from build123d import *

# Parameters (mm, degrees)
F1_DEPTH = 50
F3_DEPTH = 25
F4_R     = 4.5
F5_DEPTH = 25


with BuildPart() as f1:
    # F0 (on Top) → F1 (new body)
    with BuildSketch(Plane.XY):
        Polygon((1.597207, 5.6), (-2.124833, 5.6), (-4.124833, 5.6), (-4.124833, -6.4), (-2.124833, -6.4), (1.597207, -6.4), (3.597207, -6.4), (3.597207, 5.6), align=None)
        Polygon((-0.528539, 3), (-0.528539, 4), (0.471461, 4), (0.471461, 3), (1.597207, 3), (1.597207, -3.9), (0.471461, -3.9), (0.471461, -4.4), (-0.528539, -4.4), (-0.528539, -3.9), (-2.124833, -3.9), (-2.124833, 3), align=None, mode=Mode.SUBTRACT)
    extrude(amount=F1_DEPTH)

    # F2 (on face) → F3 (cut)
    with BuildSketch(Plane.YZ.offset(3.597207)):
        with BuildLine():
            Line((-3.9, 29.523588), (-3.9, 20.935996))
            ThreePointArc((-3.9, 20.935996), (-0.366142, 17.178962), (3.6, 20.476412))
            Line((3.6, 20.476412), (3.6, 29.064004))
            ThreePointArc((3.6, 29.064004), (0.066142, 32.821038), (-3.9, 29.523588))
        make_face()
    extrude(amount=-F3_DEPTH, mode=Mode.SUBTRACT)

    # F4 (on face) → F5 (cut)
    with BuildSketch(Plane(origin=(-4.124833, 0, 0), x_dir=(0, -1, 0), z_dir=(-1, 0, 0))):
        with Locations((0, 50)):
            Circle(F4_R)
    extrude(amount=-F5_DEPTH, mode=Mode.SUBTRACT)


solid = f1.part
Could you check a few things on this model? Use its own coordinates, in mm. A direction names the side the tool comes from. Give positions to 0.01 mm unless a question says otherwise; leave off trailing zeros. Loops run counter-clockwise (first coordinate to the right, second up) from the corner with the lowest first, then second, coordinate; pieces in that order, holes last. Notation, with made-up numbers: (-21.5, 22) -> (32.5, 22) arc R13 ccw to (32.5, 47) -> close; hole circle Ø10 at (-12, -28). An arc over 180 degrees is marked (long way). Answer as CSV lines item,"result". Start each with the question number.
(1) We'd pull the mould along Y, two halves only. Please class faces 6 (the flat face through (3.597, -4.5, 24.6)), 7 (the flat face through (0, -6.4, 25)), 8 (the flat face through (0, -4.4, 24)): released by +Y, released by -Y, zero draft, split by the parting line, or undercut.
(2) Which directions (+Z, -Z, +X, -X, +Y, -Y) give clear straight access to the entire face, cutting with the end or side of a thin tool? Please do faces 1 (the flat face through (0, 5, 50)), 2 (the flat face through (-4.125, 4, 25)), 3 (the cylindrical face through (2.404, 0.145, 32.815)), 4 (the flat face through (1, -3.9, 24)), 5 (the flat face through (1, 3, 9)).
(3) If we section it at C-C on z = 33.5: Write out the boundary of the cut face in (x, y).
(4) I need wall thicknesses on probe 1 along Y at (x, z) = (-1.75, 40); probe 2 along X at (y, z) = (-1, 11); probe 3 along Y at (x, z) = (-1.25, 29). Which ranges of each line are inside material? Lowest first, please.
(5) If we section it at B-B on x = -1: Write out the boundary of the cut face in (y, z) (3 decimals).
(6) If we section it at A-A on z = 25.5: Write out the boundary of the cut face in (x, y), then the cut area to 3 significant figures.
(7) If we section it at D-D on x = -3: Write out the boundary of the cut face in (y, z), then the cut area to 3 significant figures.
Computed:
1,face 6,"zero draft"
1,face 7,"released by -Y"
1,face 8,"undercut"
2,face 1,"+Z, +X, -X, +Y, -Y"
2,face 2,"+Z, -Z, -X, +Y, -Y"
2,face 3,"+X, -X"
2,face 4,"none"
2,face 5,"+Z, -Z"
3,outline,"(-4.12, -6.4) -> (3.6, -6.4) -> (3.6, 5.6) -> (-4.12, 5.6) -> close; hole (-2.12, -3.9) -> (-0.53, -3.9) -> (-0.53, -4.4) -> (0.47, -4.4) -> (0.47, -3.9) -> (1.6, -3.9) -> (1.6, 3) -> (0.47, 3) -> (0.47, 4) -> (-0.53, 4) -> (-0.53, 3) -> (-2.12, 3) -> close"
4,probe 1,"y = -6.4 to -3.9, 3 to 5.6"
4,probe 2,"x = -4.12 to -2.12, 1.6 to 3.6"
4,probe 3,"y = -6.4 to -3.9, 3.6 to 5.6"
5,outline,"(-6.4, 0) -> (-3.9, 0) -> (-3.9, 47.755) arc R4.5 cw to (-4.5, 50) -> (-6.4, 50) -> close; (3, 0) -> (5.6, 0) -> (5.6, 50) -> (4.5, 50) arc R4.5 cw to (3, 46.646) -> (3, 31.103) arc R3.764 cw to (3.6, 29.064) -> (3.6, 20.476) arc R3.764 cw to (3, 18.854) -> close"
6,outline,"(-4.12, -6.4) -> (3.6, -6.4) -> (3.6, -3.9) -> (0.47, -3.9) -> (0.47, -4.4) -> (-0.53, -4.4) -> (-0.53, -3.9) -> (-4.12, -3.9) -> close; (-4.12, 3.6) -> (-0.53, 3.6) -> (-0.53, 4) -> (0.47, 4) -> (0.47, 3.6) -> (3.6, 3.6) -> (3.6, 5.6) -> (-4.12, 5.6) -> close"
6,area,"33.8 mm2"
7,outline,"(-6.4, 0) -> (5.6, 0) -> (5.6, 50) -> (4.5, 50) arc R4.5 cw to (-4.5, 50) -> (-6.4, 50) -> close; hole (-3.9, 20.94) arc R3.76 ccw to (3.6, 20.48) -> (3.6, 29.06) arc R3.76 ccw to (-3.9, 29.52) -> close"
7,area,"463 mm2"
